```python
from build123d import *

# Parameters (mm, degrees)
SKETCH1_W           = 99
SKETCH1_H           = 69
BOSS_EXTRUDE1_DEPTH = 3
CUT_EXTRUDE1_DEPTH  = 2
SKETCH6_W           = 0.5
SKETCH6_H           = 1
CUT_EXTRUDE3_DEPTH  = 2
SKETCH5_W           = 17.8
SKETCH5_H           = 1
CUT_EXTRUDE2_DEPTH  = 0.5
CUT_EXTRUDE4_DEPTH  = 1.5
SKETCH8_W           = 18.8
SKETCH8_H           = 1
CUT_EXTRUDE5_DEPTH  = 0.5
SKETCH9_W           = 10
SKETCH9_H           = 10
BOSS_EXTRUDE2_DEPTH = 3
SKETCH10_R          = 1.5
CUT_EXTRUDE6_DEPTH  = 3


with BuildPart() as part:
    # Sketch1 → Boss-Extrude1 (new body)
    with BuildSketch(Plane(origin=(0, 0, 0), x_dir=(1, 0, 0), z_dir=(0, 1, 0))):
        Rectangle(SKETCH1_W, SKETCH1_H)
    extrude(amount=BOSS_EXTRUDE1_DEPTH)

    # Sketch4 → Cut-Extrude1 (cut)
    with BuildSketch(Plane(origin=(0, 3, 0), x_dir=(1, 0, 0), z_dir=(0, 1, 0))):
        Polygon((47.5, 31.149720819), (47.5, 17.443513176), (30.7, 17.443513176), (30.7, 31.149720819), (30.7, 34.5), (47.5, 34.5), align=None)
        Polygon((-47.5, 17.443513176), (-47.5, 31.149720819), (-47.5, 34.5), (-30.7, 34.5), (-30.7, 31.149720819), (-30.7, 17.443513176), align=None)
    extrude(amount=-CUT_EXTRUDE1_DEPTH, mode=Mode.SUBTRACT)

    # Sketch6 → Cut-Extrude3 (cut)
    with BuildSketch(Plane(origin=(0, 1, 0), x_dir=(1, 0, 0), z_dir=(0, 1, 0))):
        with Locations((-47.75, 31.649720819)):
            Rectangle(SKETCH6_W, SKETCH6_H)
        with Locations((-30.45, 31.649720819)):
            Rectangle(SKETCH6_W, SKETCH6_H)
        with Locations((47.75, 31.649720819)):
            Rectangle(SKETCH6_W, SKETCH6_H)
        with Locations((30.45, 31.649720819)):
            Rectangle(SKETCH6_W, SKETCH6_H)
    extrude(amount=CUT_EXTRUDE3_DEPTH, mode=Mode.SUBTRACT)

    # Sketch5 → Cut-Extrude2 (cut)
    with BuildSketch(Plane(origin=(0, 1, 0), x_dir=(1, 0, 0), z_dir=(0, 1, 0))):
        with Locations((39.1, 31.649720819)):
            Rectangle(SKETCH5_W, SKETCH5_H)
        with Locations((-39.1, 31.649720819)):
            Rectangle(SKETCH5_W, SKETCH5_H)
    extrude(amount=-CUT_EXTRUDE2_DEPTH, mode=Mode.SUBTRACT)

    # Sketch7 → Cut-Extrude4 (cut)
    with BuildSketch(Plane(origin=(0, 3, 0), x_dir=(1, 0, 0), z_dir=(0, 1, 0))):
        Polygon((-10.9, 31.149720819), (-10.9, 4.5), (6.9, 4.5), (6.9, 31.149720819), (7.4, 31.149720819), (7.4, 32.149720819), (6.9, 32.149720819), (6.9, 34.5), (-10.9, 34.5), (-10.9, 32.149720819), (-11.4, 32.149720819), (-11.4, 31.149720819), align=None)
        Polygon((8.9, 34.5), (26.7, 34.5), (26.7, 32.149720819), (27.2, 32.149720819), (27.2, 31.149720819), (26.7, 31.149720819), (26.7, 4.5), (8.9, 4.5), (8.9, 31.149720819), (8.4, 31.149720819), (8.4, 32.149720819), (8.9, 32.149720819), align=None)
    extrude(amount=-CUT_EXTRUDE4_DEPTH, mode=Mode.SUBTRACT)

    # Sketch8 → Cut-Extrude5 (cut)
    with BuildSketch(Plane(origin=(0, 1.5, 0), x_dir=(1, 0, 0), z_dir=(0, 1, 0))):
        with Locations((-2, 31.649720819)):
            Rectangle(SKETCH8_W, SKETCH8_H)
        with Locations((17.8, 31.649720819)):
            Rectangle(SKETCH8_W, SKETCH8_H)
    extrude(amount=-CUT_EXTRUDE5_DEPTH, mode=Mode.SUBTRACT)

    # Sketch9 → Boss-Extrude2 (add)
    with BuildSketch(Plane.XZ):
        with Locations((-20.8, 39.5)):
            Rectangle(SKETCH9_W, SKETCH9_H)
        with Locations((54.5, -29.5)):
            Rectangle(SKETCH9_W, SKETCH9_H)
    extrude(amount=-BOSS_EXTRUDE2_DEPTH)

    # Sketch10 → Cut-Extrude6 (cut)
    with BuildSketch(Plane(origin=(0, 3, 0), x_dir=(1, 0, 0), z_dir=(0, 1, 0))):
        with Locations(Location((-20.8, -39.5, 0), (0, 0, 270))):
            Circle(SKETCH10_R)
        with Locations(Location((54.5, 29.5, 0), (0, 0, 270))):
            Circle(SKETCH10_R)
    extrude(amount=-CUT_EXTRUDE6_DEPTH, mode=Mode.SUBTRACT)


solid = part.part
```
Geometry check sheet. Reference: the model listing, model coordinates, mm. A direction names the side the tool comes from. Give positions to 0.01 mm unless a question says otherwise; leave off trailing zeros. Order: outer loops, then holes, each group sorted by start corner. A loop starts at its lowest first (then second) coordinate and runs counter-clockwise, first axis right, second up. Notation, with made-up numbers: (-15.75, 39) -> (33.25, 39) arc R14 ccw to (33.25, 57) -> close; hole circle Ø8 at (18.5, 43). An arc over 180 degrees is marked (long way). Write each question's results on one line, items separated by ' | '. Start each with the question number.
(1) Access from +Z, -Z, +X, -X, +Y, -Y to the whole of each face (thin tool, end or side, straight path). Record for faces 4 (the face through (-25.8, 1, 39)), 5 (the face through (49.5, 1, 5)), 6 (the face through (39, 1, -24)).
(2) Scan lines: line 1 (X direction, y = 1.9, z = -9.5); line 2 (X direction, y = 1.4, z = -29.5); line 3 (X direction, y = 0.7, z = 39.5). Record each from-to range of solid material in increasing order.
(3) Sectioned sample at C-C (x = 13). Enter the section's corners in (y, z), plus the area to 4 significant figures.
(4) Gauge pin test, flat ends, axial feed: P1, Ø0.8, axis at y = 2.5, z = -16.5, coming from the +X side; P2, Ø1.6, axis at x = -38, y = 2, coming from the -Z side; P3, Ø4, axis at x = -39, z = -26.5, coming from the +Y side. Record the tip position at first contact, or that the pin passes through.
(5) Sectioned sample at D-D (z = -14). Enter the section's corners in (x, y), plus the area to 3 significant figures.
(6) Sectioned sample at A-A (x = -20.8). Enter the section's corners in (y, z).
(7) Mould release check, pull along X, two halves, no side actions. Record for faces 1 (the face through (-19.79, 1.52, 38.39)), 2 (the face through (4, 0, -3)), 3 (the face through (-15.8, 1, 39)): pulls with the +X half, pulls with the -X half, needs draft (parallel to the pull), parting line crosses it, or undercut.
(8) Sectioned sample at B-B (z = -29.5). Enter the section's corners in (x, y).
Answer below:
1) face 4: +Z, -X, +Y, -Y | face 5: +Z, +X, +Y, -Y | face 6: -Z, +Y
2) line 1: -49.5 to -10.9, 6.9 to 8.9, 26.7 to 49.5 | line 2: -49.5 to -47.5, -30.7 to 30.7, 47.5 to 53, 56 to 59.5 | line 3: -25.8 to -22.3, -19.3 to -15.8
3) outline: (0, -34.5) -> (1.5, -34.5) -> (1.5, -32.15) -> (1, -32.15) -> (1, -31.15) -> (1.5, -31.15) -> (1.5, -4.5) -> (3, -4.5) -> (3, 34.5) -> (0, 34.5) -> close | area: 161.5 mm2
4) P1: x = 49.5 | P2: z = -17.44 | P3: y = 1
5) outline: (-49.5, 0) -> (49.5, 0) -> (49.5, 3) -> (26.7, 3) -> (26.7, 1.5) -> (8.9, 1.5) -> (8.9, 3) -> (6.9, 3) -> (6.9, 1.5) -> (-10.9, 1.5) -> (-10.9, 3) -> (-49.5, 3) -> close | area: 244 mm2
6) outline: (0, -34.5) -> (3, -34.5) -> (3, 38) -> (0, 38) -> close; (0, 41) -> (3, 41) -> (3, 44.5) -> (0, 44.5) -> close
7) face 1: undercut | face 2: needs draft | face 3: pulls with the +X half
8) outline: (-49.5, 0) -> (53, 0) -> (53, 3) -> (47.5, 3) -> (47.5, 1) -> (30.7, 1) -> (30.7, 3) -> (26.7, 3) -> (26.7, 1.5) -> (8.9, 1.5) -> (8.9, 3) -> (6.9, 3) -> (6.9, 1.5) -> (-10.9, 1.5) -> (-10.9, 3) -> (-30.7, 3) -> (-30.7, 1) -> (-47.5, 1) -> (-47.5, 3) -> (-49.5, 3) -> close; (56, 0) -> (59.5, 0) -> (59.5, 3) -> (56, 3) -> close
